Check sheet for the modelled part. Datum: model origin and axes. Units: mm. Face numbers are marked on the shaded views. Round coordinates to 2 decimals unless told otherwise and drop trailing zeros. Loops run counter-clockwise (first coordinate to the right, second up) from the corner with the lowest first, then second, coordinate; pieces in that order, holes last. Notation, with made-up numbers: (49, -25.75) - (107, -25.75) arc R11 cw to (107, -18.75) - close; hole circle Ø5 at (31, -15.5). An arc over 180 degrees is marked (long way). Put each result on its own line as item: value. Start each with the question number.
Item 1: Section check B-B, the plane z = 0.55. Record the cut outline in (x, y), and give its area (3 significant figures).
Item 2: Material ranges on line 1 along Y through (x, z) = (-3, 1.9); line 2 along X through (y, z) = (-81, 3); line 3 along Z through (x, y) = (21, 2), recorded low to high.
Item 3: Section check A-A, the plane y = -6.5. Record the cut outline in (x, z).
Item 4: Gauge pin test, flat ends, axial feed: pin 1 Ø1.3 at (y, z) = (-4, 0.5) entering from +X; pin 2 Ø1.7 at (y, z) = (-3, 1) entering from -X; pin 3 Ø10 at (x, y) = (19, -25) entering from +Z. Record the tip position at first contact, or that the pin passes through.
Item 5: Draft check along Y on the marked faces 1 and 2. Enter one of: pulls with the +Y half, pulls with the -Y half, needs draft (parallel to the pull), parting line crosses it, or undercut.
Item 6: Section check D-D, the plane x = -9.5. Record the cut outline in (y, z).
Item 7: Section check C-C, the plane y = -86.5. Record the cut outline in (x, z).
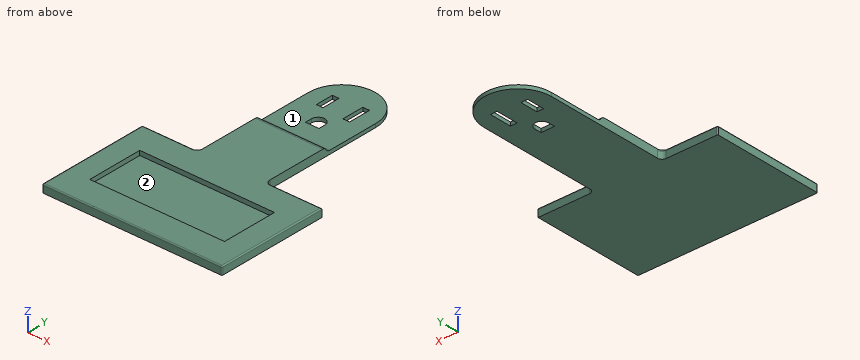
from build123d import *

# Parameters (mm, degrees)
SKETCH1_W                = 3
SKETCH1_H                = 10
SKETCH1_H_2              = 8
BOSS_EXTRUDE1_DEPTH      = 1.5875
BOSS_EXTRUDE2_DEPTH      = 40
BOSS_EXTRUDE2_DEPTH_BACK = 40
SKETCH3_W                = 2
SKETCH3_H                = 50
SKETCH3_W_2              = 1.5875
SKETCH6_W                = 2
SKETCH6_H                = 30
BOSS_EXTRUDE3_DEPTH      = 30
SKETCH4_W                = 60
SKETCH4_H                = 25
CUT_EXTRUDE1_DEPTH       = 2
FILLET3_R                = 0.5
FILLET5_R                = 2
FILLET6_R                = 2


with BuildPart() as part:
    # Sketch1 → Boss-Extrude1 (new body)
    with BuildSketch(Plane.XY):
        with BuildLine():
            Line((29.372040361, -4.693897293), (29.372040361, -59.693897293))
            Line((29.372040361, -59.693897293), (-0.627959639, -59.693897293))
            Line((-0.627959639, -59.693897293), (-0.627959639, -4.693897293))
            ThreePointArc((-0.627959639, -4.693897293), (14.372040361, 10.306102707), (29.372040361, -4.693897293))
        make_face()
        with Locations((20.722040361, -4.693897293)):
            Rectangle(SKETCH1_W, SKETCH1_H, mode=Mode.SUBTRACT)
        with Locations((8.022040361, -4.693897293)):
            Rectangle(SKETCH1_W, SKETCH1_H_2, mode=Mode.SUBTRACT)
        with BuildLine():
            ThreePointArc((17.372040361, -16.593897293), (14.372040361, -13.593897293), (11.372040361, -16.593897293))
            Line((11.372040361, -16.593897293), (11.372040361, -19.593897293))
            Line((11.372040361, -19.593897293), (17.372040361, -19.593897293))
            Line((17.372040361, -19.593897293), (17.372040361, -16.593897293))
        make_face(mode=Mode.SUBTRACT)
    extrude(amount=BOSS_EXTRUDE1_DEPTH)

    # Sketch3 → Boss-Extrude2 (add, two sides: drawn at the far end of the back side and taken through both)
    with BuildSketch(Plane(origin=(14.372040361, 0, 0), x_dir=(0, 0, -1), z_dir=(1, 0, 0)).offset(-BOSS_EXTRUDE2_DEPTH_BACK)):
        with Locations((-2.5875, -84.693897293)):
            Rectangle(SKETCH3_W, SKETCH3_H)
        with Locations((-0.79375, -84.693897293)):
            Rectangle(SKETCH3_W_2, SKETCH3_H)
    extrude(amount=BOSS_EXTRUDE2_DEPTH + BOSS_EXTRUDE2_DEPTH_BACK)

    # Sketch6 → Boss-Extrude3 (add)
    with BuildSketch(Plane(origin=(29.372040361, 0, 0), x_dir=(0, 0, -1), z_dir=(1, 0, 0))):
        with Locations((-2.5875, -44.693897293)):
            Rectangle(SKETCH6_W, SKETCH6_H)
    extrude(amount=-BOSS_EXTRUDE3_DEPTH)

    # Sketch4 → Cut-Extrude1 (cut)
    with BuildSketch(Plane.XY.offset(3.5875)):
        with Locations((14.372040361, -84.693897293)):
            Rectangle(SKETCH4_W, SKETCH4_H)
    extrude(amount=-CUT_EXTRUDE1_DEPTH, mode=Mode.SUBTRACT)

    # Fillet3
    fillet3_edges = [part.edges().sort_by_distance(p)[0] for p in [
        (-13.127959639, -59.693897293, 3.5875),
        (54.372040361, -109.693897293, 1.79375),
        (14.372040361, -109.693897293, 3.5875),
        (54.372040361, -84.693897293, 3.5875),
        (-25.627959639, -59.693897293, 1.79375),
        (-25.627959639, -109.693897293, 1.79375),
        (-25.627959639, -84.693897293, 3.5875),
        (41.872040361, -59.693897293, 3.5875),
    ]]
    fillet(fillet3_edges, radius=FILLET3_R)

    # Fillet5
    # the kernel refuses this fillet: 2 mm, written as the material it adds along each edge
    with BuildSketch(Plane(origin=(-0.627959639, -60.193897293, 3.0875), x_dir=(0, 1, 0), z_dir=(0, 0, -1))) as fillet5_piece_1_section:
        with BuildLine():
            CenterArc((0.5 + FILLET5_R, -FILLET5_R), FILLET5_R, 90, 90)
            Line((0.5 + FILLET5_R, 0), (0.5, 0))
            Line((0.5, 0), (0.5, -FILLET5_R))
        make_face()
    fillet5_piece_1 = revolve(axis=Axis((-0.627959639, -60.193897293, 3.0875), (1, 0, 0)), revolution_arc=359.64, mode=Mode.PRIVATE)
    fillet5_piece_1 = split(fillet5_piece_1, bisect_by=Plane(origin=(-1.414331511, -59.810829733, 3.5875), z_dir=(0, 0, -1)), keep=Keep.TOP, mode=Mode.PRIVATE)
    add(fillet5_piece_1)
    with BuildSketch(Plane(origin=(29.372040361, -60.193897293, 3.0875), x_dir=(0, 0.9999802608561372, -0.006283143965558423), z_dir=(0, 0.006283143965558423, 0.9999802608561372))) as fillet5_piece_2_section:
        with BuildLine():
            CenterArc((-0.5 - FILLET5_R, -FILLET5_R), FILLET5_R, 0, 90)
            Line((-0.5, -FILLET5_R), (-0.5, 0))
            Line((-0.5, 0), (-0.5 - FILLET5_R, 0))
        make_face()
    fillet5_piece_2 = revolve(axis=Axis((29.372040361, -60.193897293, 3.0875), (-1, 0, 0)), revolution_arc=359.64, mode=Mode.PRIVATE)
    fillet5_piece_2 = split(fillet5_piece_2, bisect_by=Plane(origin=(30.158412419, -59.810829718, 3.5875), z_dir=(0, 0, -1)), keep=Keep.TOP, mode=Mode.PRIVATE)
    add(fillet5_piece_2)
    with BuildSketch(Plane(origin=(29.372040361, -29.693897293, 1.5875), x_dir=(0, 0, 1), z_dir=(-1, 0, 0))) as fillet5_piece_3:
        with BuildLine():
            CenterArc((FILLET5_R, FILLET5_R), FILLET5_R, 180, 90)
            Line((0, FILLET5_R), (0, 0))
            Line((0, 0), (FILLET5_R, 0))
        make_face()
    extrude(amount=30)
    with BuildSketch(Plane(origin=(-0.627959639, -59.693897293, 3.0875), x_dir=(-1, 0, 0), z_dir=(0, 0, -1))) as fillet5_piece_4:
        with BuildLine():
            CenterArc((FILLET5_R, FILLET5_R), FILLET5_R, 180, 90)
            Line((0, FILLET5_R), (0, 0))
            Line((0, 0), (FILLET5_R, 0))
        make_face()
    extrude(amount=3.0875)
    with BuildSketch(Plane(origin=(29.372040361, -59.693897293, 0), x_dir=(0, 1, 0), z_dir=(0, 0, 1))) as fillet5_piece_5:
        with BuildLine():
            CenterArc((FILLET5_R, -FILLET5_R), FILLET5_R, 90, 90)
            Line((0, -FILLET5_R), (0, 0))
            Line((0, 0), (FILLET5_R, 0))
        make_face()
    extrude(amount=3.0875)

    # Fillet6
    fillet6_edges = [part.edges().sort_by_distance(p)[0] for p in [
        (14.372040361, -29.693897293, 3.5875),
    ]]
    fillet(fillet6_edges, radius=FILLET6_R)


solid = part.part
Check result:
1. outline: (-25.63, -109.19) arc R0.5 ccw to (-25.13, -109.69) - (53.87, -109.69) arc R0.5 ccw to (54.37, -109.19) - (54.37, -59.69) - (31.37, -59.69) arc R2 cw to (29.37, -57.69) - (29.37, -4.69) arc R15 ccw to (-0.63, -4.69) - (-0.63, -57.69) arc R2 cw to (-2.63, -59.69) - (-25.13, -59.69) arc R0.5 ccw to (-25.63, -60.19) - close; hole (6.52, -8.69) - (9.52, -8.69) - (9.52, -0.69) - (6.52, -0.69) - close; hole (11.37, -19.59) - (17.37, -19.59) - (17.37, -16.59) arc R3 ccw to (11.37, -16.59) - close; hole (19.22, -9.69) - (22.22, -9.69) - (22.22, 0.31) - (19.22, 0.31) - close
1. area: 5,920 mm²
2. line 1: -109.69 to -97.19, -72.19 to -59.69
2. line 2: -25.63 to -15.63, 44.37 to 54.37
2. line 3: 0 to 1.59
3. outline: (-0.63, 0) - (6.52, 0) - (6.52, 1.59) - (-0.63, 1.59) - close; (9.52, 0) - (19.22, 0) - (19.22, 1.59) - (9.52, 1.59) - close; (22.22, 0) - (29.37, 0) - (29.37, 1.59) - (22.22, 1.59) - close
4. pin 1: x = 29.37
4. pin 2: x = -0.6
4. pin 3: z = 3.22
5. face 1: needs draft
5. face 2: undercut
6. outline: (-109.69, 0) - (-59.69, 0) - (-59.69, 3.09) arc R0.5 ccw to (-60.19, 3.59) - (-72.19, 3.59) - (-72.19, 1.59) - (-97.19, 1.59) - (-97.19, 3.59) - (-109.19, 3.59) arc R0.5 ccw to (-109.69, 3.09) - close
7. outline: (-25.63, 0) - (54.37, 0) - (54.37, 3.09) arc R0.5 ccw to (53.87, 3.59) - (44.37, 3.59) - (44.37, 1.59) - (-15.63, 1.59) - (-15.63, 3.59) - (-25.13, 3.59) arc R0.5 ccw to (-25.63, 3.09) - close
